Verification items for the finished model (mm, model axes). Face numbers are marked on the shaded views. A direction names the side the tool comes from. Round coordinates to 2 decimals unless told otherwise and drop trailing zeros. Loops run counter-clockwise (first coordinate to the right, second up) from the corner with the lowest first, then second, coordinate; pieces in that order, holes last. Notation, with made-up numbers: M 71.5,19 L 105.5,19 A16 ccw 105.5,27 Z; hole C 22.5,16.25 d11. An arc over 180 degrees is marked long. Answer as CSV lines item,"result".
```python
from build123d import *

# Parameters (mm, degrees)
F1_W     = 10
F1_H     = 62
F4_D     = 8
F5_D     = 9.525
F7_D     = 8
F8_ANGLE = -20


# Not quite as in the source:
# - a length typed as a fraction of an inch, garbled in the dataset ("3 / 203.2 mm" for 3/8 in), is restored


with BuildPart() as f2:
    # F2: sweep along a path in F0
    with BuildLine(Plane.XY) as f2_path:
        Line((0, 0), (-113, 0))
        Line((-113, 0), (-182.5372539382, 25.3094906061))
    # F1 (on Right) → F2 (sweep)
    with BuildSketch(Plane.YZ):
        Rectangle(F1_W, F1_H)
    sweep(path=f2_path.line, transition=Transition.RIGHT)

    # F4 (through all)
    with Locations(Plane(origin=(0, 5, 0), x_dir=(-1, 0, 0), z_dir=(0, 1, 0))):
        with Locations((10, -23), (10, 23)):
            Hole(F4_D / 2)

    # F5 (through all)
    with Locations(Plane(origin=(0, 5, 0), x_dir=(-1, 0, 0), z_dir=(0, 1, 0))):
        with Locations((60, 0)):
            Hole(F5_D / 2)

    # F7 (through all)
    with Locations(Plane(origin=(-11.5083882471, -31.6190368434, 0), x_dir=(-0.9396926208, 0.3420201433, 0), z_dir=(0.3420201433, 0.9396926208, 0))):
        with Locations((117.0669010524, 20.6375), (171.0669010524, 20.6375), (171.0669010524, -20.6375), (117.0669010524, -20.6375)):
            Hole(F7_D / 2)


with BuildPart() as f2_1:
    # F8: moved
    add(f2.part.rotate(Axis((-184.2473546548, 20.6110275022, 0), (0, 0, -1)), F8_ANGLE))


solid = f2_1.part
```
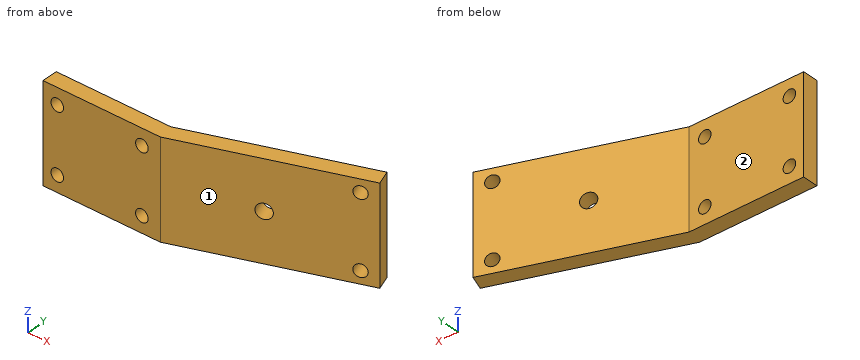
1) Section check B-B (x = -151). Record the cut outline in (y, z), plus the area to 3 significant figures.
Here are the results:
outline,"M 20.61,-31 L 30.61,-31 L 30.61,31 L 20.61,31 Z"
area,"620 mm^2"
2) Section check A-A (z = 11). Record the cut outline in (x, y), plus the area to 3 significant figures.
Here are the results:
outline,"M -184.25,20.61 L -109.37,20.61 L -2.35,59.56 L -5.77,68.96 L -111.13,30.61 L -184.25,30.61 Z"
area,"1,870 mm^2"
3) Go/stop test with flat-tipped pins: pin 1 (13 mm diameter, centred on x = -175.13, z = -20.64, fed in from +Y); pin 2 (6 mm diameter, centred on x = -110.5, z = 20, fed in from +Y). Record where each tip stops, or that it passes through.
Here are the results:
pin 1,"stops at y = 30.61"
pin 2,"stops at y = 31.93"
4) Material ranges on probe 1 along Y at (x, z) = (-161.5, -10); probe 2 along Y at (x, z) = (-45.5, -15.5), recorded low to high.
Here are the results:
probe 1,"y = 20.61 to 30.61"
probe 2,"y = 43.86 to 54.5"
5) Section check D-D (y = 53). Record the cut outline in (x, z), plus the area to 3 significant figures.
Here are the results:
outline,"M -49.62,-31 L -20.38,-31 L -20.38,31 L -49.62,31 Z"
area,"1,810 mm^2"
6) Set-up check for the marked faces 1 and 2: record each of +Z, -Z, +X, -X, +Y, -Y from which the full face is reachable in a straight line by a thin tool's end or side.
Here are the results:
face 1,"+Z, -Z, +X, -Y"
face 2,"+Z, -Z, -X, +Y"
7) Section check C-C (y = 62.5). State how many separate pieces and enclosed holes the cut face has, plus the area to 3 significant figures.
Here are the results:
separate pieces,"1"
enclosed holes,"2"
area,"1,140 mm^2"
